```python
from build123d import *

# Parameters (mm, degrees)
F0_R     = 9.525
F1_DEPTH = 49.53
F2_R     = 15.875
F2_R_2   = 9.525
F3_DEPTH = 2.54


# Not quite as in the source:
# - a fillet or chamfer that OpenCascade refuses, or shapes differently, is made with other operations: its cross-section is extruded or revolved along the edge and cut away or added


with BuildPart() as f1:
    # F0 (on Right) → F1 (new body)
    with BuildSketch(Plane.YZ):
        Circle(F0_R)
    extrude(amount=F1_DEPTH)

    # F2 (on face) → F3 (join)
    with BuildSketch(Plane.YZ.offset(49.53)):
        Circle(F2_R)
        Circle(F2_R_2, mode=Mode.SUBTRACT)
        Circle(F2_R_2)
    extrude(amount=F3_DEPTH)

    # F4: fillet of radius 12.7 on 1 edges, made by hand

    # F4_s1 → F4_t2 (revolve, cut)
    with BuildSketch(Plane.XY):
        with BuildLine():
            ThreePointArc((49.53, 15.875), (51.4182778852, 12.2710926284), (52.07, 8.255))
            Line((52.07, 8.255), (52.07, 15.875))
            Line((52.07, 15.875), (49.53, 15.875))
        make_face()
    revolve(axis=Axis((52.07, 0, 0), (1, 0, 0)), mode=Mode.SUBTRACT)


solid = f1.part
```
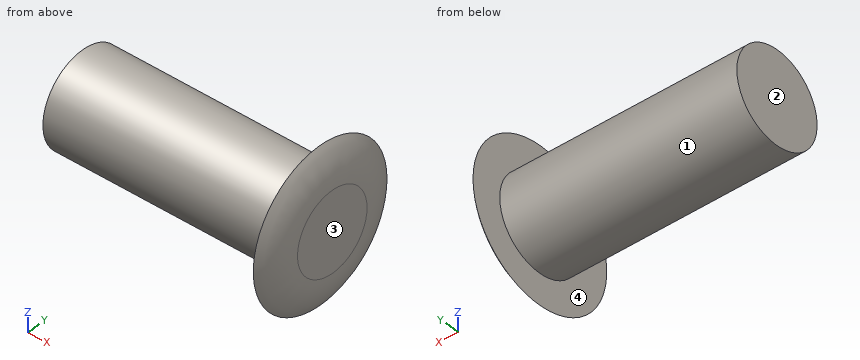
Here's how the part is built. I have some questions about the finished solid (model axes, mm). Face numbers are marked on the shaded views. A direction names the side the tool comes from. Round coordinates to 2 decimals unless told otherwise and drop trailing zeros. Order: outer loops, then holes, each group sorted by start corner. A loop starts at its lowest first (then second) coordinate and runs counter-clockwise, first axis right, second up. Notation, with made-up numbers: M -32.5,10 L 15.5,10 A30 cw 15.5,35 Z; hole C -19,-14 d11. An arc over 180 degrees is marked long. Use CSV: the item, a comma, the result in double quotes.
1) I need wall thicknesses on line 1 along X through (y, z) = (0, 8.5); line 2 along Z through (x, y) = (12, 0) (3 decimals); line 3 along Z through (x, y) = (11, -5). Which ranges of each line are inside material? Lowest first, please. Write a range as [from, to].
Taken from the geometry:
line 1,"[0, 52.07]"
line 2,"[-9.525, 9.525]"
line 3,"[-8.11, 8.11]"
2) If we mould it in two halves opening along Z, with no side actions, what happens to the marked faces 1 and 2? For each: pulls with the +Z half, pulls with the -Z half, needs draft (parallel to the pull), parting line crosses it, or undercut.
Taken from the geometry:
face 1,"parting line crosses it"
face 2,"needs draft"
3) I want a section at A-A (x = 42). List the corners of the cut face in (y, z) for me (3 decimals), then the cut area to 3 significant figures.
Taken from the geometry:
outline,"C 0,0 d19.05"
area,"285 mm^2"
4) I'm going to push flat-ended pins straight in: P1, Ø8, axis at x = 7, z = 0.5, coming from the +Y side (3 decimals); P2, Ø2, axis at y = -12, z = -8, coming from the -X side; P3, Ø12, axis at x = 44, y = -12, coming from the -Z side. Where does each tip first touch, or does it pass through?
Taken from the geometry:
P1,"y = 9.525"
P2,"x = 49.53"
P3,"z = -12.59"
5) On a 3-axis mill with a long thin cutter (end or side, diameter ignored), from which of +Z, -Z, +X, -X, +Y, -Y can I reach the whole of each face in a straight line? I mean the marked faces 3 and 4. Say none if no direction works.
Taken from the geometry:
face 3,"+Z, -Z, +X, +Y, -Y"
face 4,"-X"
